```python
from build123d import *

# Parameters (mm, degrees)
SKETCH1_W                     = 33.3
SKETCH1_H                     = 42
BOSS_EXTRUDE1_DEPTH           = 2.4
M2_5_TAPPED_HOLE1_D           = 2.05
M2_5_TAPPED_HOLE1_CSINK_D     = 2.55
M2_5_TAPPED_HOLE1_CSINK_ANGLE = 90


with BuildPart() as part:
    # Sketch1 → Boss-Extrude1 (new body)
    with BuildSketch(Plane.XY):
        with Locations((0, -7)):
            Rectangle(SKETCH1_W, SKETCH1_H)
    extrude(amount=BOSS_EXTRUDE1_DEPTH)

    # M2.5 Tapped Hole1 (through all)
    with Locations(Plane(origin=(0, 12, 0), x_dir=(-1, 0, 0), z_dir=(0, 0, -1))):
        with Locations((0, 0), (0, -6.75), (12.65, -19), (12.65, -33), (-12.65, -33), (-12.65, -19)):
            CounterSinkHole(M2_5_TAPPED_HOLE1_D / 2, M2_5_TAPPED_HOLE1_CSINK_D / 2, counter_sink_angle=M2_5_TAPPED_HOLE1_CSINK_ANGLE)


solid = part.part
```
Source: CAD feature listing. Evaluate the final solid. Frame: model axes, mm. Round coordinates to 2 decimals unless told otherwise and drop trailing zeros. Loops run counter-clockwise (first coordinate to the right, second up) from the corner with the lowest first, then second, coordinate; pieces in that order, holes last. Notation, with made-up numbers: M 17.25,-37.75 L 61.25,-37.75 A26 ccw 61.25,-8.75 Z; hole C -15.5,16.5 d11. An arc over 180 degrees is marked long. Use a Markdown table: item, result. Add a question column.
1. Cut plane A-A, the plane y = -21. Output: boundary loops of the cut face in (x, z) (3 decimals), and give its area (3 significant figures).
2. Ray query, line 1 along X through (y, z) = (-7, 1.85) (3 decimals); line 2 along Y through (x, z) = (0, 1.4) (3 decimals); line 3 along Y through (x, z) = (-12.65, 1.75) (3 decimals). Return the intervals inside material, ascending. Write a range as [from, to].
3. Pull-direction query (Y, two-part tool) for faces 1 (the flat face through (0, -7, 0)), 2 (the flat face through (0, 14, 1)), 3 (the cylindrical face through (11.837, -7.624, 1.34)); classes: +Y half, -Y half, draft (parallel to the pull), parting line (faces both ways), or undercut.
4. Contact query for a flat-ended pin moving along its axis: pin 1 (1.2 mm diameter, centred on x = -12.65, y = -7, fed in from -Z). Output: stop coordinate, or through.
5. Cut plane C-C, the plane y = 5.25. Output: boundary loops of the cut face in (x, z) (3 decimals), and give its area (3 significant figures).
6. Cut plane B-B, the plane x = -12.65. Output: boundary loops of the cut face in (y, z) (3 decimals), and give its area (3 significant figures).
Solution:
| question | item | result |
|---|---|---|
| 1 | outline | M -16.65,0 L -13.925,0 L -13.675,0.25 L -13.675,2.4 L -16.65,2.4 Z; M -11.625,0.25 L -11.375,0 L 11.375,0 L 11.625,0.25 L 11.625,2.4 L -11.625,2.4 Z; M 13.675,0.25 L 13.925,0 L 16.65,0 L 16.65,2.4 L 13.675,2.4 Z |
| 1 | area | 70.0 mm2 |
| 2 | line 1 | x = [-16.65, -13.675], [-11.625, 11.625], [13.675, 16.65] |
| 2 | line 2 | y = [-28, 4.225], [6.275, 10.975], [13.025, 14] |
| 2 | line 3 | y = [-28, -22.025], [-19.975, -8.025], [-5.975, 14] |
| 3 | face 1 | draft |
| 3 | face 2 | +Y half |
| 3 | face 3 | undercut |
| 4 | pin 1 | passes through |
| 5 | outline | M -16.65,0 L -1.275,0 L -1.025,0.25 L -1.025,2.4 L -16.65,2.4 Z; M 1.025,0.25 L 1.275,0 L 16.65,0 L 16.65,2.4 L 1.025,2.4 Z |
| 5 | area | 74.9 mm2 |
| 6 | outline | M -28,0 L -22.275,0 L -22.025,0.25 L -22.025,2.4 L -28,2.4 Z; M -19.975,0.25 L -19.725,0 L -8.275,0 L -8.025,0.25 L -8.025,2.4 L -19.975,2.4 Z; M -5.975,0.25 L -5.725,0 L 14,0 L 14,2.4 L -5.975,2.4 Z |
| 6 | area | 90.8 mm2 |
